Build history of the part. All positions in model axes, mm. A direction names the side the tool comes from. Give positions to 0.01 mm unless a question says otherwise; leave off trailing zeros. Order: outer loops, then holes, each group sorted by start corner. A loop starts at its lowest first (then second) coordinate and runs counter-clockwise, first axis right, second up. Notation, with made-up numbers: (0.5, 7) -> (43.5, 7) arc R19 cw to (43.5, 22) -> close; hole circle Ø11 at (-29, 59). An arc over 180 degrees is marked (long way). One line per question, with ' | ' between items. Start each with the question number.
(1) Cut at C-C (z = -17.5). Give the cut face in (x, y), then the cut area to 3 significant figures.
(2) Which spindle directions (+Z, -Z, +X, -X, +Y, -Y) get a long thin tool onto all of the face, cutting with end or side? Do faces 1 (the face through (33.6, -1.2, 0)), 2 (the face through (-15.95, 1.32, 1.47)), 3 (the face through (22.5, 7.1, -0.8)), 4 (the face through (-33, 1, 0)), 5 (the face through (-28, 5.6, 2)). Say none if no direction does.
(3) Drill centre lines: L1, parallel to Z at x = -15.5, y = 7.15; L2, parallel to Y at x = 27, z = 2; L3, parallel to Y at x = 19, z = -33. Where is each one in solid material? Low to high. Write a range as from..to.
(4) Cut at B-B (x = 0). Give the cut face in (y, z), then the cut area to 3 significant figures.
(5) Pull direction X, two halves, no side cores. Call faces 6 (the face through (-18, 7, -37)), 7 (the face through (16, 5.6, -4)), 8 (the face through (-10, 8.6, -8)): +X half, -X half, draft (parallel to the pull), parting line (faces both ways), or undercut.
(6) Cut at A-A (z = -2). Give the number of separate pieces and of enclosed holes in the cut face, then the cut area to 3 significant figures.
(7) Cut at D-D (y = 6.5). Give the cut face in (x, z).
(8) Pin check, flat tips, straight feed: pin 1 Ø2.5 at (x, z) = (15.5, -2) entering from +Y; pin 2 Ø1.5 at (x, y) = (22, -1) entering from -Z; pin 3 Ø2.5 at (x, z) = (31, 0.5) entering from +Y; pin 4 Ø5.5 at (x, z) = (16.5, -1) entering from -Y. Stop position of each tip, or through.
from build123d import *

# Parameters (mm, degrees)
ESBO_O1_R                = 1.6
RESSALTO_EXTRUS_O1_DEPTH = 4
ESBO_O2_W                = 42
ESBO_O2_H                = 43
ESBO_O2_R                = 13
RESSALTO_EXTRUS_O2_DEPTH = 3
CHANFRO1_SIZE            = 3
CHANFRO2_SIZE            = 5
CHANFRO3_SIZE            = 12
ESBO_O3_R                = 1.7
CORTE_EXTRUS_O1_DEPTH    = 59.060313468
ESBO_O4_R                = 3.5
CORTE_EXTRUS_O2_DEPTH    = 58.400348431
CHANFRO4_SIZE            = 8


# Some blends are built 0.0001 mm under size
with BuildPart() as part:
    # Esboço1 → Ressalto-extrusão1 (new body)
    with BuildSketch(Plane.XY):
        with BuildLine():
            Line((-35, 5.6), (35, 5.6))
            ThreePointArc((35, 5.6), (40.6, 0), (35, -5.6))
            Line((35, -5.6), (-35, -5.6))
            ThreePointArc((-35, -5.6), (-40.6, 0), (-35, 5.6))
        make_face()
        with Locations((35, 0)):
            Circle(ESBO_O1_R, mode=Mode.SUBTRACT)
        with Locations((-35, 0)):
            Circle(ESBO_O1_R, mode=Mode.SUBTRACT)
    extrude(amount=RESSALTO_EXTRUS_O1_DEPTH)

    # Esboço2 → Ressalto-extrusão2 (add)
    with BuildSketch(Plane(origin=(0, 5.6, 0), x_dir=(1, 0, 0), z_dir=(0, 1, 0))):
        with Locations((0, 17.5)):
            Rectangle(ESBO_O2_W, ESBO_O2_H)
        with Locations(Location((0, 17.5, 0), (0, 0, 180))):
            Circle(ESBO_O2_R, mode=Mode.SUBTRACT)
    extrude(amount=RESSALTO_EXTRUS_O2_DEPTH)

    # Chanfro1
    chanfro1_edges = [part.edges().sort_by_distance(p)[0] for p in [
        (21, 5.6, 2),
        (-21, 5.6, 2),
    ]]
    chamfer(chanfro1_edges, length=CHANFRO1_SIZE - 0.0001)  # a hair under: the kernel refuses the full size

    # Chanfro2
    chanfro2_edges = [part.edges().sort_by_distance(p)[0] for p in [
        (21, 7.1, -39),
        (-21, 7.1, -39),
    ]]
    chamfer(chanfro2_edges, length=CHANFRO2_SIZE)

    # Chanfro3
    # the kernel refuses this chamfer: 12 mm, written as the material it adds along each edge
    with BuildSketch(Plane(origin=(-21, 5.6, 0), x_dir=(0, 0.027495876610586417, -0.9996219169112968), z_dir=(1, 0, 0))) as chanfro3_piece_1_section:
        Polygon((CHANFRO3_SIZE * 0.999621916911, -CHANFRO3_SIZE * 0.0274958766106), (-CHANFRO3_SIZE * 0.0274958766106, -CHANFRO3_SIZE * 0.999621916911), (0, 0), align=None)
    chanfro3_piece_1 = extrude(amount=42, mode=Mode.PRIVATE)
    chanfro3_piece_1 = chanfro3_piece_1 - Plane(origin=(0, 1.3654596, -17.5), x_dir=(-1, 0, 0), z_dir=(0, -1, 0)) * Cylinder(13, 132, mode=Mode.PRIVATE)
    chanfro3_piece_1 = split(chanfro3_piece_1, bisect_by=Plane(origin=(0, -5.6, -3.473436689), z_dir=(0, 1, 0)), keep=Keep.TOP, mode=Mode.PRIVATE)
    add(chanfro3_piece_1)

    # Esboço3 → Corte-extrusão1 (cut, through all)
    with BuildSketch(Plane(origin=(0, 8.6, 0), x_dir=(1, 0, 0), z_dir=(0, 1, 0))):
        with Locations(Location((-15.5, 33, 0), (0, 0, 180))):
            Circle(ESBO_O3_R)
        with Locations(Location((15.5, 33, 0), (0, 0, 180))):
            Circle(ESBO_O3_R)
        with Locations(Location((15.5, 2, 0), (0, 0, 180))):
            Circle(ESBO_O3_R)
        with Locations(Location((-15.5, 2, 0), (0, 0, 224.900872156))):
            Circle(ESBO_O3_R)
    extrude(amount=-CORTE_EXTRUS_O1_DEPTH, mode=Mode.SUBTRACT)

    # Esboço4 → Corte-extrusão2 (cut, through all)
    with BuildSketch(Plane.XZ.offset(-5.6)):
        with Locations(Location((-15.5, -2, 0), (0, 0, 159.948957433))):
            Circle(ESBO_O4_R)
        with Locations(Location((15.5, -2, 0), (0, 0, 159.948957433))):
            Circle(ESBO_O4_R)
        with Locations((15.5, -33)):
            Circle(ESBO_O4_R)
        with Locations((-15.5, -33)):
            Circle(ESBO_O4_R)
    extrude(amount=CORTE_EXTRUS_O2_DEPTH, mode=Mode.SUBTRACT)

    # Chanfro4
    # the kernel refuses this chamfer: 8 mm, written as the material it adds along each edge
    with BuildSketch(Plane(origin=(21, 29.173363904, 0), x_dir=(-0.027495876610586494, 3.1525903256593395e-13, -0.9996219169112968), z_dir=(0, -1, 0))) as chanfro4_piece_1_section:
        Polygon((CHANFRO4_SIZE * 0.999621916911, CHANFRO4_SIZE * 0.0274958766106), (-CHANFRO4_SIZE * 0.0274958766106, CHANFRO4_SIZE * 0.999621916911), (0, 0), align=None)
    chanfro4_piece_1 = extrude(amount=34.773363904, mode=Mode.PRIVATE)
    chanfro4_piece_1 = split(chanfro4_piece_1, bisect_by=Plane(origin=(26.011530684, 3.588369316, -1.04435595), z_dir=(0.7071067811865474, 0.7071067811865478, 0)), keep=Keep.TOP, mode=Mode.PRIVATE)
    chanfro4_piece_1 = split(chanfro4_piece_1, bisect_by=Plane(origin=(26.682074245, 5.6, -1.04435595), z_dir=(0, -1, 0)), keep=Keep.TOP, mode=Mode.PRIVATE)
    add(chanfro4_piece_1)
    with BuildSketch(Plane(origin=(21, 29.173363904, 0), x_dir=(-0.027495876610586494, 3.1525903256593395e-13, -0.9996219169112968), z_dir=(0, -1, 0))) as chanfro4_piece_2_section:
        Polygon((CHANFRO4_SIZE * 0.999621916911, CHANFRO4_SIZE * 0.0274958766106), (-CHANFRO4_SIZE * 0.0274958766106, CHANFRO4_SIZE * 0.999621916911), (0, 0), align=None)
    chanfro4_piece_2 = extrude(amount=34.773363904, mode=Mode.PRIVATE)
    chanfro4_piece_2 = split(chanfro4_piece_2, bisect_by=Plane(origin=(22.348256975, 7.251643025, -3.639481653), z_dir=(-0.7071067811865474, -0.7071067811865478, 0)), keep=Keep.TOP, mode=Mode.PRIVATE)
    chanfro4_piece_2 = split(chanfro4_piece_2, bisect_by=Plane(origin=(21.792799579, 8.6, -3.639481653), z_dir=(0, -1, 0)), keep=Keep.TOP, mode=Mode.PRIVATE)
    chanfro4_piece_2 = split(chanfro4_piece_2, bisect_by=Plane(origin=(21.792799579, 5.6, -3.639481653), z_dir=(0, 1, 0)), keep=Keep.TOP, mode=Mode.PRIVATE)
    add(chanfro4_piece_2)
    with BuildSketch(Plane(origin=(21, 29.173363904, 0), x_dir=(-0.027495876610586494, 3.1525903256593395e-13, -0.9996219169112968), z_dir=(0, -1, 0))) as chanfro4_piece_3_section:
        Polygon((CHANFRO4_SIZE * 0.999621916911, CHANFRO4_SIZE * 0.0274958766106), (-CHANFRO4_SIZE * 0.0274958766106, CHANFRO4_SIZE * 0.999621916911), (0, 0), align=None)
    chanfro4_piece_3 = extrude(amount=34.773363904, mode=Mode.PRIVATE)
    chanfro4_piece_3 = split(chanfro4_piece_3, bisect_by=Plane(origin=(23.6247191, -1.786159604, -4.613840396), z_dir=(0, 0.7071067811862648, 0.7071067811868302)), keep=Keep.TOP, mode=Mode.PRIVATE)
    chanfro4_piece_3 = split(chanfro4_piece_3, bisect_by=Plane(origin=(26.361426714, 3.238473286, -2.325915119), z_dir=(-0.7071067811865474, -0.7071067811865478, 0)), keep=Keep.TOP, mode=Mode.PRIVATE)
    chanfro4_piece_3 = split(chanfro4_piece_3, bisect_by=Plane(origin=(23.6247191, 5.6, -2.325915119), z_dir=(0, -1, 0)), keep=Keep.TOP, mode=Mode.PRIVATE)
    add(chanfro4_piece_3)
    with BuildSketch(Plane(origin=(-21, -5.6, 0), x_dir=(0.027495876610578507, 3.1525903256593415e-13, -0.999621916911297), z_dir=(0, 1, 0))) as chanfro4_piece_4_section:
        Polygon((CHANFRO4_SIZE * 0.999621916911, CHANFRO4_SIZE * 0.0274958766106), (-CHANFRO4_SIZE * 0.0274958766111, CHANFRO4_SIZE * 0.999621916911), (0, 0), align=None)
    chanfro4_piece_4 = extrude(amount=34.773363904, mode=Mode.PRIVATE)
    chanfro4_piece_4 = split(chanfro4_piece_4, bisect_by=Plane(origin=(-23.6247191, -1.786159604, -4.613840396), z_dir=(0, 0.7071067811862648, 0.7071067811868302)), keep=Keep.TOP, mode=Mode.PRIVATE)
    chanfro4_piece_4 = split(chanfro4_piece_4, bisect_by=Plane(origin=(-26.361426714, 3.238473286, -2.325915119), z_dir=(0.7071067811865477, -0.7071067811865475, 0)), keep=Keep.TOP, mode=Mode.PRIVATE)
    chanfro4_piece_4 = split(chanfro4_piece_4, bisect_by=Plane(origin=(-23.6247191, 5.6, -2.325915119), z_dir=(0, -1, 0)), keep=Keep.TOP, mode=Mode.PRIVATE)
    add(chanfro4_piece_4)
    with BuildSketch(Plane(origin=(-21, -5.6, 0), x_dir=(0.027495876610578507, 3.1525903256593415e-13, -0.999621916911297), z_dir=(0, 1, 0))) as chanfro4_piece_5_section:
        Polygon((CHANFRO4_SIZE * 0.999621916911, CHANFRO4_SIZE * 0.0274958766106), (-CHANFRO4_SIZE * 0.0274958766111, CHANFRO4_SIZE * 0.999621916911), (0, 0), align=None)
    chanfro4_piece_5 = extrude(amount=34.773363904, mode=Mode.PRIVATE)
    chanfro4_piece_5 = split(chanfro4_piece_5, bisect_by=Plane(origin=(-26.011530684, 3.588369316, -1.04435595), z_dir=(-0.7071067811865477, 0.7071067811865475, 0)), keep=Keep.TOP, mode=Mode.PRIVATE)
    chanfro4_piece_5 = split(chanfro4_piece_5, bisect_by=Plane(origin=(-26.682074245, 5.6, -1.04435595), z_dir=(0, -1, 0)), keep=Keep.TOP, mode=Mode.PRIVATE)
    add(chanfro4_piece_5)
    with BuildSketch(Plane(origin=(-21, -5.6, 0), x_dir=(0.027495876610578507, 3.1525903256593415e-13, -0.999621916911297), z_dir=(0, 1, 0))) as chanfro4_piece_6_section:
        Polygon((CHANFRO4_SIZE * 0.999621916911, CHANFRO4_SIZE * 0.0274958766106), (-CHANFRO4_SIZE * 0.0274958766111, CHANFRO4_SIZE * 0.999621916911), (0, 0), align=None)
    chanfro4_piece_6 = extrude(amount=34.773363904, mode=Mode.PRIVATE)
    chanfro4_piece_6 = split(chanfro4_piece_6, bisect_by=Plane(origin=(-22.348256975, 7.251643025, -3.639481653), z_dir=(0.7071067811865477, -0.7071067811865475, 0)), keep=Keep.TOP, mode=Mode.PRIVATE)
    chanfro4_piece_6 = split(chanfro4_piece_6, bisect_by=Plane(origin=(-21.792799579, 8.6, -3.639481653), z_dir=(0, -1, 0)), keep=Keep.TOP, mode=Mode.PRIVATE)
    chanfro4_piece_6 = split(chanfro4_piece_6, bisect_by=Plane(origin=(-21.792799579, 5.6, -3.639481653), z_dir=(0, 1, 0)), keep=Keep.TOP, mode=Mode.PRIVATE)
    add(chanfro4_piece_6)


solid = part.part
Result set:
1) outline: (-21, 5.6) -> (-13, 5.6) -> (-13, 8.6) -> (-21, 8.6) -> close; (13, 5.6) -> (21, 5.6) -> (21, 8.6) -> (13, 8.6) -> close | area: 48.0 mm2
2) face 1: -Z, +X, +Y, -Y | face 2: -Y | face 3: +Z, -Z, +X, +Y | face 4: -Z, -X, +Y, -Y | face 5: +Z, -Z, -X, +Y
3) L1: z = -39..-34.7, -31.3..-3.7, -0.3..4 | L2: y = -5.6..5.6 | L3: y = 5.6..8.6
4) outline: (-5.6, -0.8) -> (-1.9, -4.5) -> (8.6, -4.5) -> (8.6, 4) -> (-5.6, 4) -> close; (5.6, -39) -> (8.6, -39) -> (8.6, -30.5) -> (5.6, -30.5) -> close | area: 139 mm2
5) face 6: -X half | face 7: undercut | face 8: draft
6) separate pieces: 3 | enclosed holes: 0 | area: 515 mm2
7) outline: (-23.1, -5.9) -> (-21, -8) -> (-21, -34) -> (-16, -39) -> (16, -39) -> (21, -34) -> (21, -8) -> (23.1, -5.9) -> (23.1, 4) -> (-23.1, 4) -> close; hole circle Ø3.4 at (-15.5, -33); hole circle Ø3.4 at (-15.5, -2); hole circle Ø26 at (0, -17.5); hole circle Ø3.4 at (15.5, -33); hole circle Ø3.4 at (15.5, -2)
8) pin 1: passes through | pin 2: stops at z = -6.15 | pin 3: stops at y = 5.6 | pin 4: stops at y = -5.6
